from build123d import *

# Parameters (mm, degrees)
BOSS_EXTRUDE1_DEPTH = 3.175


with BuildPart() as part:
    # Sketch1 → Boss-Extrude1 (new body)
    with BuildSketch(Plane(origin=(0, 0, 0), x_dir=(1, 0, 0), z_dir=(0, 1, 0))):
        with BuildLine():
            Line((0, 26.67), (3.175, 26.67))
            Line((3.175, 26.67), (3.175, 47.625))
            Line((3.175, 47.625), (13.97, 47.625))
            Line((13.97, 47.625), (13.97, 50.8))
            Line((13.97, 50.8), (24.13, 50.8))
            Line((24.13, 50.8), (24.13, 47.625))
            Line((24.13, 47.625), (34.925, 47.625))
            ThreePointArc((34.925, 47.625), (26.259844873, 19.005936751), (3.175, 0))
            Line((3.175, 0), (3.175, 11.43))
            Line((3.175, 11.43), (0, 11.43))
            Line((0, 11.43), (0, 26.67))
        make_face()
    extrude(amount=BOSS_EXTRUDE1_DEPTH)


solid = part.part
Geometry: final body of the model. Coordinates: model frame, mm. A direction names the side the tool comes from. Give positions to 0.01 mm unless a question says otherwise; leave off trailing zeros. Loops run counter-clockwise (first coordinate to the right, second up) from the corner with the lowest first, then second, coordinate; pieces in that order, holes last. Notation, with made-up numbers: M 76,7 L 121,7 A24 cw 121,30 Z; hole C 79,11 d9. An arc over 180 degrees is marked long. Put each result on its own line as item: value.
1) Cut plane C-C, the plane z = -13. Return the cut outline in (x, y) (3 decimals).
Computed values:
outline: M 0,0 L 21.581,0 L 21.581,3.175 L 0,3.175 Z
2) First-contact query: P1, Ø1, axis at x = 7.5, y = 1.5, coming from the +Z side; P2, Ø1.6, axis at y = 1, z = -38, coming from the -X side (3 decimals); P3, Ø1.6, axis at y = 1, z = -48.5, coming from the -X side. Flat tips, straight axial feed; report the tip coordinate or a pass-through.
Computed values:
P1: stops at z = -1.78
P2: stops at x = 3.175
P3: stops at x = 13.97
3) Material intervals for L1, parallel to X at y = 2.7, z = -26.5; L2, parallel to Z at x = 21, y = 2.9; L3, parallel to X at y = 2.75, z = -11 (3 decimals), sorted ascending. Write a range as from..to.
Computed values:
L1: x = 0..30.4
L2: z = -50.8..-12.37
L3: x = 3.175..19.67
4) Cut plane B-B, the plane x = 8. Return the cut outline in (y, z) (3 decimals).
Computed values:
outline: M 0,-47.625 L 3.175,-47.625 L 3.175,-2.311 L 0,-2.311 Z
5) Cut plane A-A, the plane y = 1.25. Return the cut outline in (x, z) (1 decimal), plus the area to 3 significant figures.
Computed values:
outline: M 0,-26.7 L 3.2,-26.7 L 3.2,-47.6 L 14,-47.6 L 14,-50.8 L 24.1,-50.8 L 24.1,-47.6 L 34.9,-47.6 A51.6 ccw 3.2,0 L 3.2,-11.4 L 0,-11.4 Z
area: 1,170 mm^2
6) Reachability of faces 1 (the flat face through (2, 2, -11.43)), 2 (the flat face through (19, 2, -50.8)), 3 (the flat face through (8, 2, -47.625)), 4 (the flat face through (29, 2, -47.625)) from +Z, -Z, +X, -X, +Y, -Y: full face, straight path, thin tool, end or side. Return the list, or none.
Computed values:
face 1: +Z, -X, +Y, -Y
face 2: -Z, +X, -X, +Y, -Y
face 3: -Z, -X, +Y, -Y
face 4: -Z, +X, +Y, -Y
